from build123d import *

# Parameters (mm, degrees)
F0_W     = 20
F0_H     = 91
F1_DEPTH = 60
F2_T     = 2.5
F4_DEPTH = 25.001


with BuildPart() as f1:
    # F0 (on Top) → F1 (new body)
    with BuildSketch(Plane.XY):
        Rectangle(F0_W, F0_H)
    extrude(amount=F1_DEPTH)

    # F2
    f2_openings = [f1.faces().sort_by_distance(p)[0] for p in [
        (0, 0, 60),
    ]]
    offset(amount=F2_T, openings=f2_openings, kind=Kind.INTERSECTION)

    # F3 (on face) → F4 (cut, through all)
    with BuildSketch(Plane.YZ.offset(12.5)):
        with BuildLine():
            ThreePointArc((-12.5, 60), (0, 47.5), (12.5, 60))
            Line((12.5, 60), (-12.5, 60))
        make_face()
    extrude(amount=-F4_DEPTH, mode=Mode.SUBTRACT)


solid = f1.part
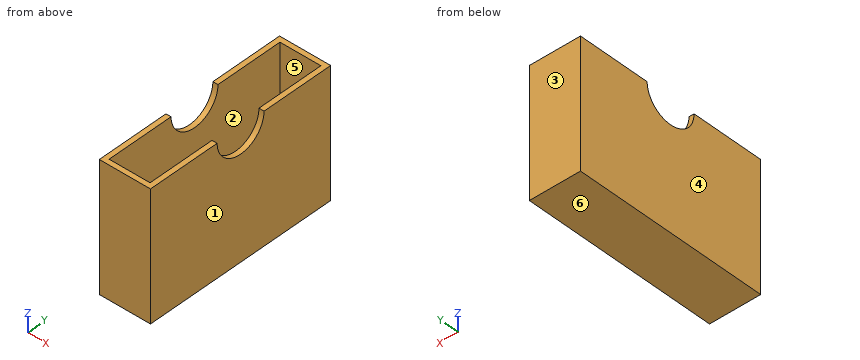
Can you work these out from the model? Positions are in its coordinate system, mm. Face numbers are marked on the shaded views. A direction names the side the tool comes from. Coordinates: 2 decimals unless noted, no trailing zeros. Write each loop counter-clockwise with the first axis right and the second up, starting at its lowest first coordinate (ties: lowest second). Pieces come first, ordered by that corner, then holes. Notation, with made-up numbers: M -13,-19.5 L 1,-19.5 A33 ccw 1,18.5 Z; hole C 75,-36.5 d2. An arc over 180 degrees is marked long. Use one line per item in the form item = value.
Q1. If we section it at A-A (z = 24): Write out the boundary of the cut face in (x, y).
Model answer:
outline = M -12.5,-48 L 12.5,-48 L 12.5,48 L -12.5,48 Z; hole M -10,-45.5 L 10,-45.5 L 10,45.5 L -10,45.5 Z
Q2. We'd pull the mould along X, two halves only. Please class the marked faces 1, 2, 3 and 4: +X half, -X half, draft (parallel to the pull), parting line (faces both ways), or undercut.
Model answer:
face_1 = +X half
face_2 = undercut
face_3 = draft
face_4 = -X half
Q3. For the marked faces 5 and 6, which set-ups out of +Z, -Z, +X, -X, +Y, -Y let a thin tool reach every point of the face, with its end or its side?
Model answer:
face_5 = +Z
face_6 = -Z, +X, -X, +Y, -Y
Q4. If we section it at D-D (y = -37.5): Write out the boundary of the cut face in (x, z), then the cut area to 4 significant figures.
Model answer:
outline = M -12.5,-2.5 L 12.5,-2.5 L 12.5,60 L 10,60 L 10,0 L -10,0 L -10,60 L -12.5,60 Z
area = 362.5 mm^2
Q5. If we section it at C-C (x = -0.75): Write out the boundary of the cut face in (y, z).
Model answer:
outline = M -48,-2.5 L 48,-2.5 L 48,60 L 45.5,60 L 45.5,0 L -45.5,0 L -45.5,60 L -48,60 Z
Q6. For P1, Ø6, axis at x = 3.5, y = 8.5, coming from the +Z side, with a flat end and sliding along its axis, tell me the tip position at first contact or that it passes through.
Model answer:
P1 = 0
Q7. If we section it at B-B (z = 55): Write out the boundary of the cut face in (x, y), then the cut area to 3 significant figures.
Model answer:
outline = M -12.5,-48 L 12.5,-48 L 12.5,-11.46 L 10,-11.46 L 10,-45.5 L -10,-45.5 L -10,-11.46 L -12.5,-11.46 Z; M -12.5,11.46 L -10,11.46 L -10,45.5 L 10,45.5 L 10,11.46 L 12.5,11.46 L 12.5,48 L -12.5,48 Z
area = 465 mm^2
Q8. I need wall thicknesses on line 1 along Y through (x, z) = (6, 29); line 2 along X through (y, z) = (3, 47); line 3 along Z through (x, y) = (-1.5, 28). Which ranges of each line are inside material? Lowest first, please. Write a range as from..to.
Model answer:
line_1 = -48..-45.5, 45.5..48
line_2 = -12.5..-10, 10..12.5
line_3 = -2.5..0
